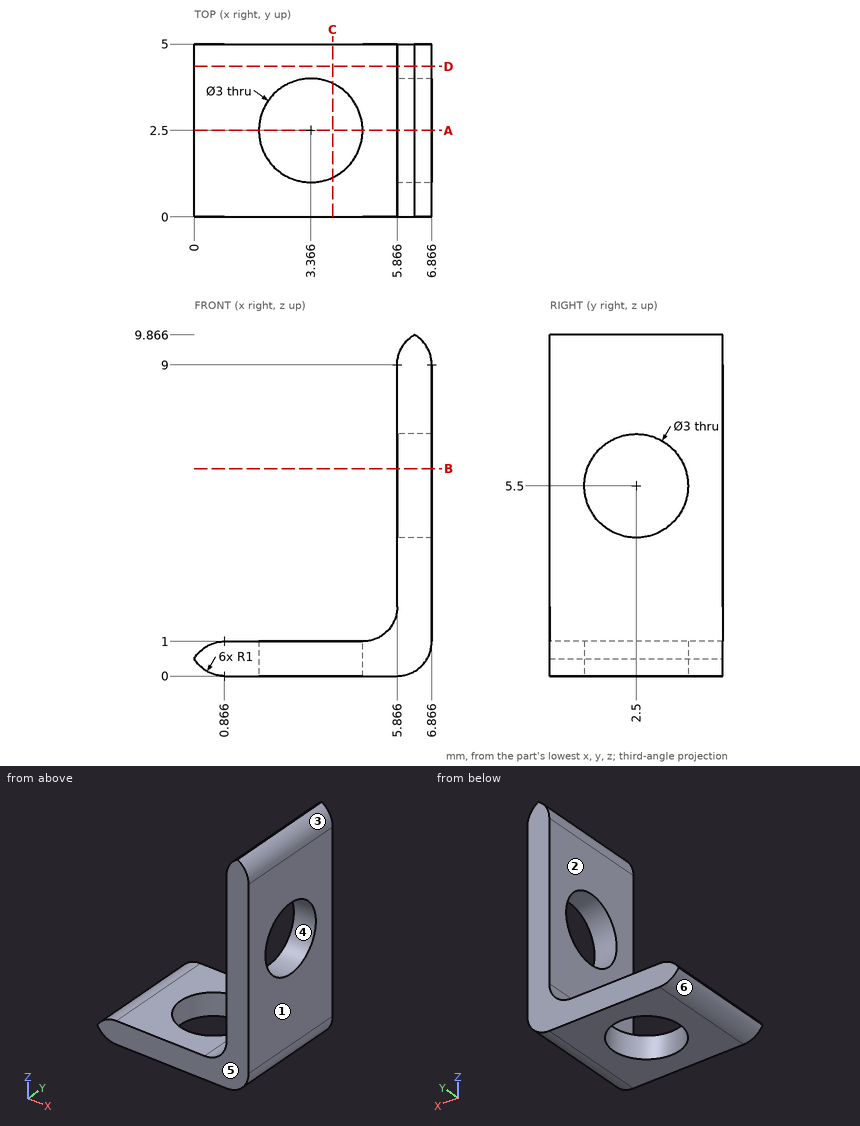
Verification items for this drawing (mm, ordinates from the low corner). A direction names the side the tool comes from. Coordinates: 2 decimals unless noted, no trailing zeros. Loops run counter-clockwise (first coordinate to the right, second up) from the corner with the lowest first, then second, coordinate; pieces in that order, holes last. Notation, with made-up numbers: (59.25, -1) - (80.25, -1) arc R8 ccw to (80.25, 12) - close; hole circle Ø3 at (-29.75, 79). An arc over 180 degrees is marked (long way). Answer as a JSON object with one key per item and string values.
(1) Cross-section at D-D, the plane y = 4.35. Record the boundary of the cut face in (x, z), then the cut area to 3 significant figures.
Response:
{"outline": "(0, 0.5) arc R1 ccw to (0.87, 0) - (5.87, 0) arc R1 ccw to (6.87, 1) - (6.87, 9) arc R1 ccw to (6.37, 9.87) arc R1 ccw to (5.87, 9) - (5.87, 2) arc R1 cw to (4.87, 1) - (0.87, 1) arc R1 ccw to start", "area": "15.2 mm²"}
(2) Cross-section at C-C, the plane x = 4. Record the boundary of the cut face in (y, z).
Response:
{"outline": "(0, 0) - (1.14, 0) - (1.14, 1) - (0, 1) - close; (3.86, 0) - (5, 0) - (5, 1) - (3.86, 1) - close"}
(3) Cross-section at A-A, the plane y = 2.5. Count the separate pieces of the cut face and the enclosed holes in it.
Response:
{"separate pieces": "3", "enclosed holes": "0"}
(4) Mould release check, pull along Z, two halves, no side actions. Record for the marked faces 3, 4, 5 and 6: pulls with the +Z half, pulls with the -Z half, needs draft (parallel to the pull), parting line crosses it, or undercut.
Response:
{"face 3": "pulls with the +Z half", "face 4": "undercut", "face 5": "needs draft", "face 6": "pulls with the -Z half"}
(5) Cross-section at B-B, the plane z = 6. Record the boundary of the cut face in (x, y).
Response:
{"outline": "(5.87, 0) - (6.87, 0) - (6.87, 1.09) - (5.87, 1.09) - close; (5.87, 3.91) - (6.87, 3.91) - (6.87, 5) - (5.87, 5) - close"}
(6) Go/stop test with flat-tipped pins: pin 1 Ø3 at (y, z) = (3, 4.5) entering from -X; pin 2 Ø1.8 at (x, y) = (3.37, 2.5) entering from +Z; pin 3 Ø1 at (x, y) = (1, 2.5) entering from +Z. Record where each tip stops, or that it passes through.
Response:
{"pin 1": "stops at x = 5.87", "pin 2": "passes through", "pin 3": "stops at z = 1"}
(7) Access from +Z, -Z, +X, -X, +Y, -Y to the whole of each face (thin tool, end or side, straight path). Record for the marked faces 1 and 2.
Response:
{"face 1": "+Z, -Z, +X, +Y, -Y", "face 2": "+Z, -X, +Y, -Y"}
(8) Scan lines: line 1 along Z through (x, y) = (1.5, 0.4); line 2 along X through (y, z) = (4.4, 3.5); line 3 along Z through (x, y) = (6.15, 2.5). Record each from-to range of solid material in increasing order.
Response:
{"line 1": "z = 0 to 1", "line 2": "x = 5.87 to 6.87", "line 3": "z = 0.04 to 4, 7 to 9.7"}
